Autodesk Inventor part; units mm, degrees
ref_plane "YZ Plane" through (0, 0, 0) normal (1, 0, 0) x (0, 1, 0)
ref_plane "XZ Plane" through (0, 0, 0) normal (0, 1, 0) x (-1, 0, 0)
ref_plane "XY Plane" through (0, 0, 0) normal (0, 0, 1) x (1, 0, 0)
sketch "Sketch1" plane through (0, 0, 0) normal (0, 0, 1) x (1, 0, 0)
  line L0 (4.0654, 27.1063) -> (2.3055, 18.8848)
  line L1 (2.3055, 18.8848) -> (-5.6945, 16.2981)
  line L2 (-5.6945, 16.2981) -> (-11.9346, 21.933)
  line L3 (-11.9346, 21.933) -> (-10.1748, 30.1545)
  line L4 (-10.1748, 30.1545) -> (-2.1748, 32.7412)
  line L5 (-2.1748, 32.7412) -> (4.0654, 27.1063)
  circle A0 centre (-3.9346, 24.5196) radius 3.5
extrude "Extrusion4" add sketch "Sketch1" against normal blind 5
sketch "Sketch2" plane through (0, 0, 0) normal (0, 0, 1) x (1, 0, 0)
  point P0 (0, 0)
properties part number "gaica" material "Bronze, Soft Tin"
Part model, mm, in its own coordinate system. Coordinates: 2 decimals unless noted, no trailing zeros. Loops run counter-clockwise (first coordinate to the right, second up) from the corner with the lowest first, then second, coordinate; pieces in that order, holes last. Notation, with made-up numbers: (26, 50.25) -> (32, 50.25) arc R28 ccw to (32, 68.25) -> close; hole circle Ø3 at (51, 37.5). An arc over 180 degrees is marked (long way). Use a Markdown table: item, result. Add a question column.
Item 1: Band-saw the part on C-C on z = -3.2. Write the cut outline in (x, y).
Item 2: Pull direction Y, two halves, no side cores. Call faces 1 (the flat face through (-8, 25, 0)), 2 (the flat face through (-1.64, 17.61, -2.46)), 3 (the cylindrical face through (-4.39, 27.99, -2.46)): +Y half, -Y half, draft (parallel to the pull), parting line (faces both ways), or undercut.
Item 3: Band-saw the part on D-D on y = 28.5. Write the cut outline in (x, z), plus the area to 3 significant figures.
Item 4: Probe probe 1 along X at (y, z) = (24.75, -2.65); probe 2 along X at (y, z) = (22, -4.4); probe 3 along Y at (x, z) = (-2.5, -2.6). List the from-to ranges inside material, lowest first.
Item 5: Band-saw the part on B-B on x = -2.5. Write the cut outline in (y, z), plus the area to 3 significant figures.
Item 6: Band-saw the part on A-A on y = 24. Write the cut outline in (x, z).
Item 7: Flat gauge pins, fed straight in: P1, Ø3, axis at x = 2, z = -1, coming from the -Y side; P2, Ø1, axis at y = 18.5, z = -3.5, coming from the -X side; P3, Ø8, axis at x = -7, y = 20.5, coming from the +Z side; P4, Ø1, axis at x = -4.5, z = -4, coming from the +Y side. Where does each tip first touch, or does it go through?
Geometry says:
| question | item | result |
|---|---|---|
| 1 | outline | (-11.93, 21.93) -> (-5.69, 16.3) -> (2.31, 18.88) -> (4.07, 27.11) -> (-2.17, 32.74) -> (-10.17, 30.15) -> close; hole circle Ø7 at (-3.93, 24.52) |
| 2 | face 1 | draft |
| 2 | face 2 | -Y half |
| 2 | face 3 | undercut |
| 3 | outline | (-10.53, -5) -> (2.52, -5) -> (2.52, 0) -> (-10.53, 0) -> close |
| 3 | area | 65.3 mm² |
| 4 | probe 1 | -11.33 to -7.43, -0.44 to 3.56 |
| 4 | probe 2 | -11.92 to -6.36, -1.51 to 2.97 |
| 4 | probe 3 | 17.33 to 21.33, 27.71 to 32.64 |
| 5 | outline | (17.33, -5) -> (21.33, -5) -> (21.33, 0) -> (17.33, 0) -> close; (27.71, -5) -> (32.64, -5) -> (32.64, 0) -> (27.71, 0) -> close |
| 5 | area | 44.6 mm² |
| 6 | outline | (-11.49, -5) -> (-7.4, -5) -> (-7.4, 0) -> (-11.49, 0) -> close; (-0.47, -5) -> (3.4, -5) -> (3.4, 0) -> (-0.47, 0) -> close |
| 7 | P1 | y = 18.3 |
| 7 | P2 | x = -8.69 |
| 7 | P3 | z = 0 |
| 7 | P4 | y = 32.15 |
